Source: CAD feature listing. Evaluate the final solid. Frame: model axes, mm. A direction names the side the tool comes from. Give positions to 0.01 mm unless a question says otherwise; leave off trailing zeros. Write each loop counter-clockwise with the first axis right and the second up, starting at its lowest first coordinate (ties: lowest second). Pieces come first, ordered by that corner, then holes. Notation, with made-up numbers: (-24, -23) - (5, -23) arc R29 ccw to (5, 0) - close; hole circle Ø1 at (76, -6). An arc over 180 degrees is marked (long way). One line per question, with ' | ' between items. Start each with the question number.
(1) Draft query along Z for faces 5 (the flat face through (18, -6.68, 10)), 6 (the cylindrical face through (5.08, -0.79, 21.11)), 7 (the cylindrical face through (27.94, -5.67, 15.37)). Return one class per face: +Z half, -Z half, draft (parallel to the pull), parting line (faces both ways), or undercut.
(2) Section C-C, the plane z = 3.75. Return loops of the section in (x, y), plus the area to 3 significant figures.
(3) Ray query, line 1 (Z direction, x = 17.5, y = -4.5) (3 decimals); line 2 (Z direction, x = 41, y = -1); line 3 (Y direction, x = 23, z = 3). Return the intervals inside material, ascending. Write a range as [from, to].
(4) Access query for faces 1 (the flat face through (12.7, -4, 10)), 2 (the flat face through (81.407, -4, 23)), 3 (the flat face through (43.307, -6, 15)), 4 (the flat face through (52.197, -6, 15)). Directions: +Z, -Z, +X, -X, +Y, -Y. A direction counts if a zero-diameter tool reaches every point of the face in a straight line with its end or side. Return the directions, or none.
(5) Pin query (flat end, axial travel): pin 1 (5 mm diameter, centred on x = 87.5, z = 11, fed in from -Y); pin 2 (4.5 mm diameter, centred on x = 34.5, y = -6, fed in from +Z); pin 3 (5 mm diameter, centred on x = 92, y = -3, fed in from +Z). Return the tip coordinate at first contact, or that it passes through.
(6) Section A-A, the plane y = -3.75. State how many separate pieces and enclosed holes the cut face has, plus the area to 3 significant figures.
(7) Section B-B, the plane x = 17. Return loops of the section in (y, z) (3 decimals).
(8) Section D-D, the plane x = 64. Return loops of the section in (y, z), plus the area to 3 significant figures.
```python
from build123d import *

# Parameters (mm, degrees)
F0_W     = 122.047
F0_H     = 25.146
F0_R     = 1.778
F1_DEPTH = 1.6002
F2_W     = 10.16
F2_H     = 8.89
F2_W_2   = 13.97
F2_H_2   = 6.35
F3_DEPTH = 5.08
F4_W     = 8.89
F4_H     = 8.89
F4_R     = 2.8575
F4_W_2   = 5.715
F4_H_2   = 5.715
F5_DEPTH = 8.255


with BuildPart() as f1:
    # F0 (on Front) → F1 (new body)
    with BuildSketch(Plane.XZ):
        with Locations((61.0235, 12.573)):
            Rectangle(F0_W, F0_H)
        with Locations((6.858, 21.0312)):
            Circle(F0_R, mode=Mode.SUBTRACT)
        with BuildLine():
            ThreePointArc((113.157, 19.2532), (111.379, 21.0312), (113.157, 22.8092))
            Line((113.157, 22.8092), (117.094, 22.8092))
            ThreePointArc((117.094, 22.8092), (118.872, 21.0312), (117.094, 19.2532))
            Line((117.094, 19.2532), (113.157, 19.2532))
        make_face(mode=Mode.SUBTRACT)
    extrude(amount=F1_DEPTH)

    # F2 (on face) → F3 (join)
    with BuildSketch(Plane.XZ.offset(1.6002)):
        with Locations((17.78, 10.16)):
            Rectangle(F2_W, F2_H)
        with Locations((74.422, 23.241)):
            Rectangle(F2_W_2, F2_H_2)
    extrude(amount=F3_DEPTH)

    # F4 (on face) → F5 (join)
    with BuildSketch(Plane.XZ.offset(1.6002)):
        with Locations((47.752, 14.605)):
            Rectangle(F4_W, F4_H)
        with Locations((82.677, 5.08)):
            Circle(F4_R)
        with Locations((33.655, 15.3035)):
            Rectangle(F4_W_2, F4_H_2)
        with BuildLine():
            Line((30.7975, 12.446), (30.7975, 18.161))
            ThreePointArc((30.7975, 18.161), (27.94, 15.3035), (30.7975, 12.446))
        make_face()
        with BuildLine():
            ThreePointArc((36.5125, 12.446), (39.37, 15.3035), (36.5125, 18.161))
            Line((36.5125, 18.161), (36.5125, 12.446))
        make_face()
    extrude(amount=F5_DEPTH)


solid = f1.part
```
Check sheet entries:
1) face 5: draft | face 6: undercut | face 7: parting line
2) outline: (0, -1.6) - (80.15, -1.6) - (80.15, -9.86) - (85.21, -9.86) - (85.21, -1.6) - (122.05, -1.6) - (122.05, 0) - (0, 0) - close | area: 237 mm²
3) line 1: [5.715, 14.605] | line 2: [0, 25.15] | line 3: [-1.6, 0]
4) face 1: +Z, -Z, -X, -Y | face 2: +Z, +X, -Y | face 3: +Z, -Z, -Y | face 4: +Z, -Z, +X, -Y
5) pin 1: y = -1.6 | pin 2: z = 18.16 | pin 3: z = 25.15
6) separate pieces: 5 | enclosed holes: 0 | area: 342 mm²
7) outline: (-6.68, 5.715) - (-1.6, 5.715) - (-1.6, 0) - (0, 0) - (0, 25.146) - (-1.6, 25.146) - (-1.6, 14.605) - (-6.68, 14.605) - close
8) outline: (-1.6, 0) - (0, 0) - (0, 25.15) - (-1.6, 25.15) - close | area: 40.2 mm²
